The figure shows three views and two pictorial views of one solid part (mm, origin at its lowest corner). Answer the questions. Coordinates: 2 decimals unless noted, no trailing zeros. Loops run counter-clockwise (first coordinate to the right, second up) from the corner with the lowest first, then second, coordinate; pieces in that order, holes last. Notation, with made-up numbers: M -11.5,87 L 0.5,87 A15 ccw 0.5,103 Z; hole C 84,24.25 d1. An arc over 180 degrees is marked long. Write each question's results on one line, items separated by ' | '.
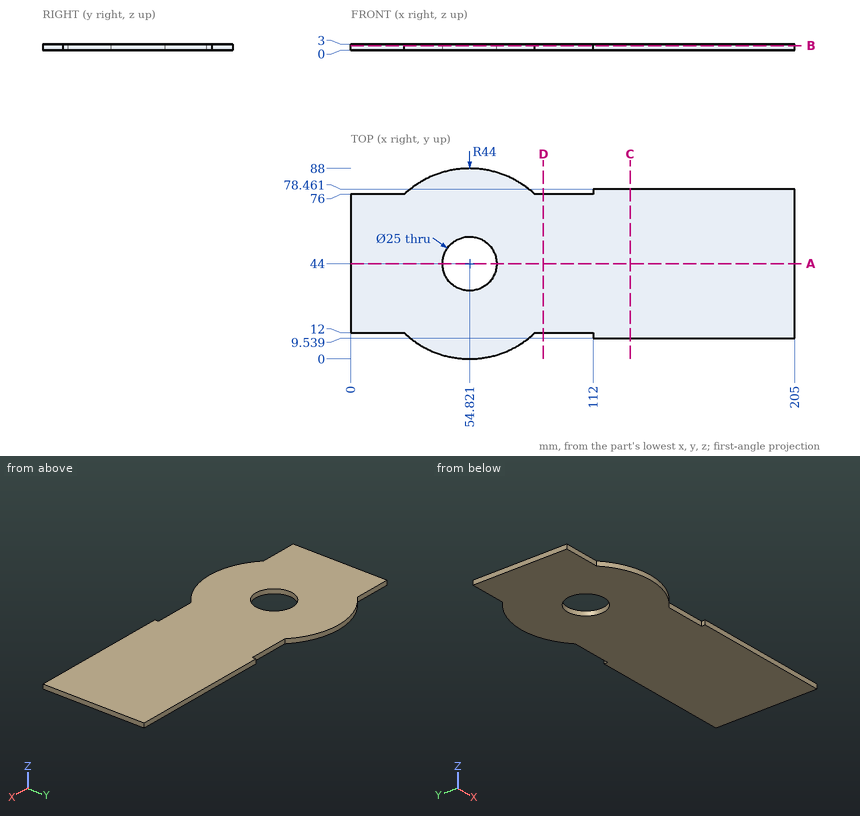
1) Find section D-D, the plane x = 89. Give the vertices of the cut face in (y, z).
Check result:
outline: M 12,0 L 76,0 L 76,3 L 12,3 Z
2) Find section B-B, the plane z = 2.25. Give the vertices of the cut face in (x, y).
Check result:
outline: M 0,12 L 24.62,12 A44 ccw 85.02,12 L 112,12 L 112,9.54 L 205,9.54 L 205,78.46 L 112,78.46 L 112,76 L 85.02,76 A44 ccw 24.62,76 L 0,76 Z; hole C 54.82,44 d25
3) Find section C-C, the plane x = 129. Give the vertices of the cut face in (y, z).
Check result:
outline: M 9.54,0 L 78.46,0 L 78.46,3 L 9.54,3 Z
4) Given pin 1 Ø1 at (x, z) = (137.5, 0.5) entering from +Y; pin 2 Ø0.9 at (x, z) = (167.5, 1.5) entering from -Y; pin 3 Ø1.5 at (x, z) = (96.5, 2) entering from +Y; pin 4 Ø6 at (x, y) = (91.5, 62.5) entering from -Z, each flat-ended and moving along its own axis, determine where each tip first touches the part or whether it passes through.
Check result:
pin 1: y = 78.46 | pin 2: y = 9.54 | pin 3: y = 76 | pin 4: z = 0
5) Find section A-A, the plane y = 44. Give the vertices of the cut face in (x, z).
Check result:
outline: M 0,0 L 42.32,0 L 42.32,3 L 0,3 Z; M 67.32,0 L 205,0 L 205,3 L 67.32,3 Z
6) Straight lines are drawn through the part: probe 1 along X at (y, z) = (44, 0.8); probe 2 along Y at (x, z) = (55, 0.3); probe 3 along Y at (x, z) = (16, 0.75). For each, find the intervals that lie inside material, in ascending order. Write a range as [from, to].
Check result:
probe 1: [0, 42.32], [67.32, 205] | probe 2: [0, 31.5], [56.5, 88] | probe 3: [12, 76]
